Can you work these out from the model? Positions are in its coordinate system, mm. A direction names the side the tool comes from. Give positions to 0.01 mm unless a question says otherwise; leave off trailing zeros. Loops run counter-clockwise (first coordinate to the right, second up) from the corner with the lowest first, then second, coordinate; pieces in that order, holes last. Notation, with made-up numbers: M 25.5,-21 L 29.5,-21 A9 cw 29.5,-6 Z; hole C -1.5,-24.5 d7. An arc over 180 degrees is marked long. Answer as a JSON object with one key per item and string values.
```python
from build123d import *

# Parameters (mm, degrees)
F0_R     = 6.86
F1_DEPTH = 10
F2_R     = 2.5
F3_DEPTH = 11.501


with BuildPart() as f1:
    # F0 (on Top) → F1 (new body)
    with BuildSketch(Plane.XY):
        with BuildLine():
            Line((3, -14.952987), (3, -7.952987))
            ThreePointArc((3, -7.952987), (0, 8.5), (-3, -7.952987))
            Line((-3, -7.952987), (-3, -14.952987))
            Line((-3, -14.952987), (-1.6, -14.952987))
            Line((-1.6, -14.952987), (-1.6, -8))
            Line((-1.6, -8), (1.6, -8))
            Line((1.6, -8), (1.6, -14.952987))
            Line((1.6, -14.952987), (3, -14.952987))
        make_face()
        Circle(F0_R, mode=Mode.SUBTRACT)
    extrude(amount=F1_DEPTH)

    # F2 (on face) → F3 (cut, through all)
    with BuildSketch(Plane(origin=(-3, 0, 0), x_dir=(0, -1, 0), z_dir=(-1, 0, 0))):
        with Locations((11.452987, 5)):
            Circle(F2_R)
    extrude(amount=-F3_DEPTH, mode=Mode.SUBTRACT)


solid = f1.part
```
1) Suppose I cut it at B-B, the plane x = 0. Write out the boundary of the cut face in (y, z), and give its area (3 significant figures).
Answer list:
{"outline": "M -8,0 L -6.86,0 L -6.86,10 L -8,10 Z; M 6.86,0 L 8.5,0 L 8.5,10 L 6.86,10 Z", "area": "27.8 mm^2"}
2) If we mould it in two halves opening along Z, with no side actions, what happens to faces 1 (the cylindrical face through (-2.31, -8.955, 5.11)), 2 (the flat face through (2, -14.953, 5)), 3 (the flat face through (2, -7, 10))? For each: +Z half, -Z half, draft (parallel to the pull), parting line (faces both ways), or undercut.
Answer list:
{"face 1": "undercut", "face 2": "draft", "face 3": "+Z half"}
3) For faces 4 (the flat face through (3, -14, 4)), 5 (the flat face through (0, -8, 5)), 6 (the flat face through (-3, -14, 4)), which set-ups out of +Z, -Z, +X, -X, +Y, -Y let a thin tool reach every point of the face, with its end or its side?
Answer list:
{"face 4": "+Z, -Z, +X, -Y", "face 5": "+Z, -Z, -Y", "face 6": "+Z, -Z, -X, -Y"}
4) Will these pins go through, and if not, where does the flat tip stop? pin 1 Ø6 at (x, z) = (-6.5, 8.5) entering from -Y; pin 2 Ø3.5 at (y, z) = (-10, 4) entering from +X; pin 3 Ø4 at (x, y) = (-1, -5.5) entering from +Z; pin 4 Ø4 at (y, z) = (-11.45, 5) entering from -X.
Answer list:
{"pin 1": "y = -7.75", "pin 2": "x = 3", "pin 3": "z = 10", "pin 4": "through"}
5) Please list where these lines run through material, in increasing order: line 1 along X through (y, z) = (-10, 8.5); line 2 along Y through (x, z) = (-2.5, 8.75); line 3 along X through (y, z) = (-3.5, 2). Write a range as from..to.
Answer list:
{"line 1": "-3..-1.6, 1.6..3", "line 2": "-14.95..-6.39, 6.39..8.12", "line 3": "-7.75..-5.9, 5.9..7.75"}
6) Suppose I cut it at C-C, the plane y = 0. Write out the boundary of the cut face in (x, z).
Answer list:
{"outline": "M -8.5,0 L -6.86,0 L -6.86,10 L -8.5,10 Z; M 6.86,0 L 8.5,0 L 8.5,10 L 6.86,10 Z"}
7) Suppose I cut it at A-A, the plane z = 5. Write out the boundary of the cut face in (x, y).
Answer list:
{"outline": "M -3,-14.95 L -1.6,-14.95 L -1.6,-13.95 L -3,-13.95 Z; M -3,-8.95 L -1.6,-8.95 L -1.6,-8 L 1.6,-8 L 1.6,-8.95 L 3,-8.95 L 3,-7.95 A8.5 ccw long -3,-7.95 Z; M 1.6,-14.95 L 3,-14.95 L 3,-13.95 L 1.6,-13.95 Z; hole C 0,0 d13.72"}
8) Suppose I cut it at D-D, the plane z = 1. Write out the boundary of the cut face in (x, y), and give its area (3 significant figures).
Answer list:
{"outline": "M -3,-14.95 L -1.6,-14.95 L -1.6,-8 L 1.6,-8 L 1.6,-14.95 L 3,-14.95 L 3,-7.95 A8.5 ccw long -3,-7.95 Z; hole C 0,0 d13.72", "area": "96.7 mm^2"}
